Source: CAD feature listing. Evaluate the final solid. Frame: model axes, mm. A direction names the side the tool comes from. Give positions to 0.01 mm unless a question says otherwise; leave off trailing zeros. Order: outer loops, then holes, each group sorted by start corner. A loop starts at its lowest first (then second) coordinate and runs counter-clockwise, first axis right, second up. Notation, with made-up numbers: M 71,-33 L 102,-33 A25 cw 102,-11 Z; hole C 77.25,70.25 d11. An arc over 180 degrees is marked long. Answer in a Markdown table with one row per item. Add a question column.
(1) Section query C-C, the plane z = 29. Return loops of the section in (x, y), plus the area to 3 significant figures.
(2) Section query A-A, the plane y = 0. Return loops of the section in (x, z), plus the area to 3 significant figures.
(3) Material intervals for line 1 along Z through (x, y) = (-87, 8); line 2 along Z through (x, y) = (38.5, 86.5); line 3 along Z through (x, y) = (64, -46), sorted ascending.
(4) Section query B-B, the plane x = 7. Return loops of the section in (y, z), plus the area to 3 significant figures.
(5) Mould query, pull axis Y, two halves, no side actions, for faces 4 (the face through (82.79, -61.55, 21.7)), 5 (the face through (2.68, 88.96, 67.99)), 6 (the face through (88.998, 0.641, 0.986)). Classes: pulls with the +Y half, pulls with the -Y half, needs draft (parallel to the pull), parting line crosses it, or undercut.
(6) Section query D-D, the plane y = 76.5. Return loops of the section in (x, z).
(7) Set-up query: faces 1 (the face through (-1.2, 88.99, 0.99)), 2 (the face through (24, 58, 36)), 3 (the face through (-75, -10, 61.833)). Return all of +Z, -Z, +X, -X, +Y, -Y with unobstructed straight access to the full face (end or side cutting, diameter ignored); none if empty.
(8) Pin query (flat end, axial travel): P1, Ø12, axis at y = 61, z = 22, coming from the +X side; P2, Ø1, axis at x = -58.5, z = 23.5, coming from the +Y side; P3, Ø10, axis at x = 32, z = 39, coming from the -Y side. Return the tip coordinate at first contact, or that it passes through.
from build123d import *

# Parameters (mm, degrees)
F2_DEPTH  = 2
F4_DEPTH  = 65
F6_DEPTH  = 2
F8_DEPTH  = 25
F9_DEPTH  = 120
F11_DEPTH = 69.001


with BuildPart() as f2:
    # F1 (on face) → F2 (new body)
    with BuildSketch(Plane.XY):
        with BuildLine():
            ThreePointArc((-74.296702, -49), (0, 89), (74.296702, -49))
            Line((74.296702, -49), (71, -52))
            Line((71, -52), (63, -54))
            Line((63, -54), (63, -69.461646))
            Line((63, -69.461646), (78.302185, -65.6361))
            Line((78.302185, -65.6361), (85.728307, -58.878327))
            ThreePointArc((85.728307, -58.878327), (0, 104), (-85.728307, -58.878327))
            Line((-85.728307, -58.878327), (-78.302185, -65.6361))
            Line((-78.302185, -65.6361), (-63, -69.461646))
            Line((-63, -69.461646), (-63, -54))
            Line((-63, -54), (-71, -52))
            Line((-71, -52), (-74.296702, -49))
        make_face()
    extrude(amount=F2_DEPTH)

    # F3 (on face) → F4 (join)
    with BuildSketch(Plane.XY.offset(2)):
        with BuildLine():
            Line((-78.302185, -65.6361), (-63, -69.461646))
            Line((-63, -69.461646), (63, -69.461646))
            Line((63, -69.461646), (78.302185, -65.6361))
            Line((78.302185, -65.6361), (85.728307, -58.878327))
            ThreePointArc((85.728307, -58.878327), (0, 104), (-85.728307, -58.878327))
            Line((-85.728307, -58.878327), (-78.302185, -65.6361))
        make_face()
    extrude(amount=F4_DEPTH)

    # F5 (on face) → F6 (join)
    with BuildSketch(Plane.XY.offset(67)):
        with BuildLine():
            Line((63, -54), (71, -52))
            Line((71, -52), (74.296702, -49))
            ThreePointArc((74.296702, -49), (0, 89), (-74.296702, -49))
            Line((-74.296702, -49), (-71, -52))
            Line((-71, -52), (-63, -54))
            Line((-63, -54), (-63, -69.461646))
            Line((-63, -69.461646), (63, -69.461646))
            Line((63, -69.461646), (63, -54))
        make_face()
    extrude(amount=F6_DEPTH)

    # F7 (on face) → F8 (cut)
    with BuildSketch(Plane.XZ.offset(69.461646)):
        Polygon((88.5, 56.833451), (88.5, 61.833451), (-88.5, 61.833451), (-88.5, 56.833451), (-85.443249, 56.833451), (-85.443249, 53.333451), (-82.8, 53.333451), (-77.27866, -2), (77.27866, -2), (82.8, 53.333451), (85.443249, 53.333451), (85.443249, 56.833451), align=None)
    extrude(amount=F8_DEPTH, mode=Mode.SUBTRACT)

    # F7 (on face) → F9 (cut)
    with BuildSketch(Plane.XZ.offset(69.461646)):
        Polygon((88.5, 56.833451), (88.5, 61.833451), (-88.5, 61.833451), (-88.5, 56.833451), (-85.443249, 56.833451), (-85.443249, 53.333451), (-82.8, 53.333451), (-77.27866, -2), (77.27866, -2), (82.8, 53.333451), (85.443249, 53.333451), (85.443249, 56.833451), align=None)
    extrude(amount=-F9_DEPTH, mode=Mode.SUBTRACT)

    # F10 (on face) → F11 (cut, through all)
    with BuildSketch(Plane.XY.offset(69)):
        Polygon((-63, -4), (-63, -54), (-63, -69.461646), (0, -69.461646), (63, -69.461646), (63, -54), (63, -4), (48, 48), (0, 68), (-48, 48), align=None)
    extrude(amount=-F11_DEPTH, mode=Mode.SUBTRACT)


solid = f2.part
Values follow:
| question | item | result |
|---|---|---|
| 1 | outline | M -85.73,-58.88 L -80.37,-63.75 L -80.37,50.54 L -41.91,50.54 L 0,68 L 41.91,50.54 L 80.37,50.54 L 80.37,-63.75 L 85.73,-58.88 A104 ccw long Z |
| 1 | area | 10,300 mm² |
| 2 | outline | M -104,0 L -89,0 L -89,2 L -77.68,2 L -82.8,53.33 L -85.44,53.33 L -85.44,56.83 L -88.5,56.83 L -88.5,61.83 L -61.85,61.83 L -61.85,69 L -89,69 L -89,67 L -104,67 Z; M 61.85,61.83 L 88.5,61.83 L 88.5,56.83 L 85.44,56.83 L 85.44,53.33 L 82.8,53.33 L 77.68,2 L 89,2 L 89,0 L 104,0 L 104,67 L 89,67 L 89,69 L 61.85,69 Z |
| 2 | area | 3,330 mm² |
| 3 | line 1 | z = 2 to 56.83, 61.83 to 69 |
| 3 | line 2 | z = 0 to 67 |
| 3 | line 3 | z = 61.83 to 69 |
| 4 | outline | M 65.08,2 L 88.72,2 L 88.72,0 L 103.76,0 L 103.76,67 L 88.72,67 L 88.72,69 L 65.08,69 Z |
| 4 | area | 2,590 mm² |
| 5 | face 4 | pulls with the -Y half |
| 5 | face 5 | parting line crosses it |
| 5 | face 6 | undercut |
| 6 | outline | M -70.45,0 L -45.48,0 L -45.48,2 L 45.48,2 L 45.48,0 L 70.45,0 L 70.45,67 L 45.48,67 L 45.48,69 L -45.48,69 L -45.48,67 L -70.45,67 Z |
| 7 | face 1 | -Z, -Y |
| 7 | face 2 | +Z, -Z, -Y |
| 7 | face 3 | -Y |
| 8 | P1 | stops at x = 88.27 |
| 8 | P2 | stops at y = 86.32 |
| 8 | P3 | stops at y = 52.58 |
